from build123d import *

# Parameters (mm, degrees)
SKETCH1_W                       = 82.55
SKETCH1_H                       = 120.65
BOSS_EXTRUDE1_DEPTH             = 69.85
SKETCH2_W                       = 76.2
SKETCH2_H                       = 25.4
CUT_EXTRUDE1_DEPTH              = 107.95
SKETCH3_W                       = 5.08
SKETCH3_H                       = 101.6
CUT_EXTRUDE2_DEPTH              = 8.89
SKETCH4_W                       = 63.5
SKETCH4_H                       = 19.05
CUT_EXTRUDE3_DEPTH              = 83.55
SKETCH5_W                       = 57.15
SKETCH5_H                       = 25.4
CUT_EXTRUDE4_DEPTH              = 121.65
F_40_0_138_DIAMETER_HOLE1_D     = 3.5052
F_40_0_138_DIAMETER_HOLE1_DEPTH = 13.97
BOSS_EXTRUDE2_DEPTH             = 6.35
SKETCH15_W                      = 57.15
SKETCH15_H                      = 88.9
CUT_EXTRUDE5_DEPTH              = 12.7
SKETCH16_W                      = 69.85
SKETCH16_H                      = 6.35
CUT_EXTRUDE6_DEPTH              = 83.55
SKETCH17_R                      = 1.7526
CUT_EXTRUDE7_DEPTH              = 6.35


with BuildPart() as part:
    # Sketch1 → Boss-Extrude1 (new body)
    with BuildSketch(Plane.XY):
        with Locations((0, 79.375)):
            Rectangle(SKETCH1_W, SKETCH1_H)
    extrude(amount=BOSS_EXTRUDE1_DEPTH)

    # Sketch2 → Cut-Extrude1 (cut)
    with BuildSketch(Plane(origin=(0, 139.7, 0), x_dir=(1, 0, 0), z_dir=(0, 1, 0))):
        with Locations((0, -43.18)):
            Rectangle(SKETCH2_W, SKETCH2_H)
    extrude(amount=-CUT_EXTRUDE1_DEPTH, mode=Mode.SUBTRACT)

    # Sketch3 → Cut-Extrude2 (cut)
    with BuildSketch(Plane.XY.offset(69.85)):
        with Locations((30.48, 69.85)):
            Rectangle(SKETCH3_W, SKETCH3_H)
    cut_extrude2 = extrude(amount=-CUT_EXTRUDE2_DEPTH, mode=Mode.SUBTRACT)

    # Mirror1: Cut-Extrude2 across plane
    add(cut_extrude2.mirror(Plane(origin=(0, 0, 0), x_dir=(0, 0, 1), z_dir=(1, 0, 0))), mode=Mode.SUBTRACT)

    # Sketch4 → Cut-Extrude3 (cut, through all)
    with BuildSketch(Plane.ZY.offset(41.275)):
        with Locations((38.1, 130.175)):
            Rectangle(SKETCH4_W, SKETCH4_H)
    extrude(amount=-CUT_EXTRUDE3_DEPTH, mode=Mode.SUBTRACT)

    # Sketch5 → Cut-Extrude4 (cut, through all)
    with BuildSketch(Plane(origin=(0, 139.7, 0), x_dir=(1, 0, 0), z_dir=(0, 1, 0))):
        with Locations((0, -12.7)):
            Rectangle(SKETCH5_W, SKETCH5_H)
    extrude(amount=-CUT_EXTRUDE4_DEPTH, mode=Mode.SUBTRACT)

    # #40 (0.138) Diameter Hole1
    with Locations(Plane.XY.offset(69.85)):
        with Locations((-24.130002345, 92.720002179), (24.129997606, 91.450000321), (8.889995651, 40.650000908)):
            Hole(F_40_0_138_DIAMETER_HOLE1_D / 2, depth=F_40_0_138_DIAMETER_HOLE1_DEPTH)

    # Sketch14 → Boss-Extrude2 (add)
    with BuildSketch(Plane.XZ.offset(-19.05)):
        Polygon((-41.275, 69.85), (-33.02, 69.85), (-33.02, 60.96), (-27.94, 60.96), (-27.94, 69.85), (27.94, 69.85), (27.94, 60.96), (33.02, 60.96), (33.02, 69.85), (41.275, 69.85), (41.275, 0), (28.575, 0), (28.575, 25.4), (-28.575, 25.4), (-28.575, 0), (-41.275, 0), align=None)
    extrude(amount=BOSS_EXTRUDE2_DEPTH)

    # Sketch15 → Cut-Extrude5 (cut)
    with BuildSketch(Plane(origin=(0, 0, 25.4), x_dir=(-1, 0, 0), z_dir=(0, 0, -1))):
        with Locations((0, 57.15)):
            Rectangle(SKETCH15_W, SKETCH15_H)
    extrude(amount=-CUT_EXTRUDE5_DEPTH, mode=Mode.SUBTRACT)

    # Sketch16 → Cut-Extrude6 (cut, through all)
    with BuildSketch(Plane(origin=(41.275, 0, 0), x_dir=(0, 0, -1), z_dir=(1, 0, 0))):
        with Locations((-34.925, 15.875)):
            Rectangle(SKETCH16_W, SKETCH16_H)
    extrude(amount=-CUT_EXTRUDE6_DEPTH, mode=Mode.SUBTRACT)

    # Sketch17 → Cut-Extrude7 (cut)
    with BuildSketch(Plane.XY.offset(6.35)):
        with Locations((-34.925, 133.35)):
            Circle(SKETCH17_R)
    cut_extrude7 = extrude(amount=-CUT_EXTRUDE7_DEPTH, mode=Mode.SUBTRACT)

    # Mirror2: Cut-Extrude7 across plane
    add(cut_extrude7.mirror(Plane(origin=(0, 0, 0), x_dir=(0, 0, 1), z_dir=(1, 0, 0))), mode=Mode.SUBTRACT)


solid = part.part
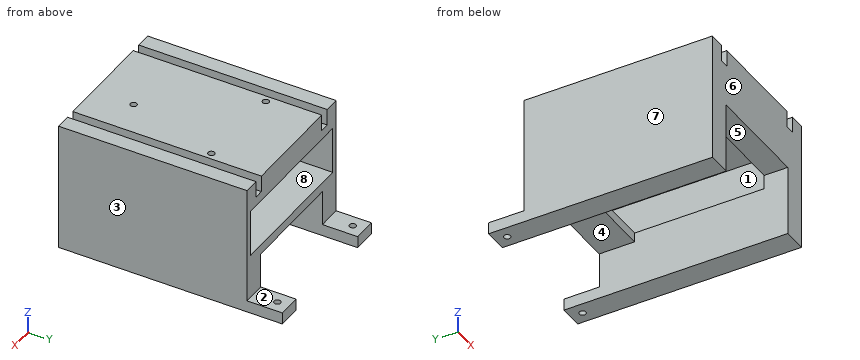
For this review, take the finished solid that the model builds, in its own axes (mm). Face numbers are marked on the shaded views. A direction names the side the tool comes from. Give positions to 0.01 mm unless a question says otherwise; leave off trailing zeros. Order: outer loops, then holes, each group sorted by start corner. A loop starts at its lowest first (then second) coordinate and runs counter-clockwise, first axis right, second up. Notation, with made-up numbers: (46, 89) - (71, 89) arc R25 cw to (71, 102) - close; hole circle Ø2 at (26, 5). An arc over 180 degrees is marked (long way). Answer as a JSON object with one key per item and string values. Group by question number.
Item 1: Take a section at D-D on z = 22.5. Give the boundary of the cut face in (x, y) (3 decimals).
Item 2: Machinability: for the marked faces 1, 2, 3 and 4, which of the approach directions +Z, -Z, +X, -X, +Y, -Y give a long, thin tool a straight path to every point of the face, cutting with its end or side? Answer none if there is none.
Item 3: Take a section at A-A on z = 5. Give the boundary of the cut face in (x, y) (3 decimals).
Item 4: Take a section at B-B on x = 0.5. Give the boundary of the cut face in (y, z), and give its area (3 significant figures).
Item 5: Draft analysis for pull direction X (two halves, no side actions). For the marked faces 5, 6, 7 and 8, state which applies: pulls with the +X half, pulls with the -X half, needs draft (parallel to the pull), parting line crosses it, or undercut.
Item 6: Wall thickness on line 1 along X through (y, z) = (133.35, 4) (3 decimals); line 2 along X through (y, z) = (43, 64.5) (3 decimals); line 3 along Z through (x, y) = (29, 114): over which ranges is each line inside the solid? List them lowest first.
Item 7: Clearance check with flat-ended pins moving along their axes: pin 1 Ø10 at (x, y) = (-32.5, 128.5) entering from +Z; pin 2 Ø19 at (x, z) = (-3.5, 32) entering from +Y; pin 3 Ø1.5 at (x, z) = (-8.5, 27) entering from -Y. State where each tip first meets the part, or that it passes through.
Item 8: Take a section at C-C on y = 40.65. Give the boundary of the cut face in (x, z) (3 decimals), and give its area (3 significant figures).
Reported:
{
 "1": {"outline": "(-41.275, 19.05) - (-28.575, 19.05) - (-28.575, 120.65) - (-41.275, 120.65) - close; (28.575, 19.05) - (41.275, 19.05) - (41.275, 120.65) - (28.575, 120.65) - close"},
 "2": {"face 1": "+Y", "face 2": "+Z, +X, -X, +Y", "face 3": "+Z, -Z, +X, +Y, -Y", "face 4": "-Z, +Y, -Y"},
 "3": {"outline": "(-41.275, 19.05) - (-28.575, 19.05) - (-28.575, 139.7) - (-41.275, 139.7) - close; (28.575, 19.05) - (41.275, 19.05) - (41.275, 139.7) - (28.575, 139.7) - close; hole circle Ø3.505 at (-34.925, 133.35); hole circle Ø3.505 at (34.925, 133.35)"},
 "4": {"outline": "(19.05, 38.1) - (31.75, 38.1) - (31.75, 55.88) - (120.65, 55.88) - (120.65, 69.85) - (19.05, 69.85) - close; (101.6, 25.4) - (120.65, 25.4) - (120.65, 30.48) - (101.6, 30.48) - close", "area": "1,740 mm^2"},
 "5": {"face 5": "undercut", "face 6": "needs draft", "face 7": "pulls with the -X half", "face 8": "undercut"},
 "6": {"line 1": "-41.275 to -36.678, -33.172 to -28.575, 28.575 to 33.172, 36.678 to 41.275", "line 2": "-41.275 to -33.02, -27.94 to 27.94, 33.02 to 41.275", "line 3": "0 to 30.48, 55.88 to 60.96"},
 "7": {"pin 1": "z = 6.35", "pin 2": "y = 120.65", "pin 3": "y = 101.6"},
 "8": {"outline": "(-41.275, 0) - (-28.575, 0) - (-28.575, 30.48) - (-38.1, 30.48) - (-38.1, 55.88) - (7.137, 55.88) - (7.137, 69.85) - (-27.94, 69.85) - (-27.94, 60.96) - (-33.02, 60.96) - (-33.02, 69.85) - (-41.275, 69.85) - close; (10.643, 55.88) - (38.1, 55.88) - (38.1, 30.48) - (28.575, 30.48) - (28.575, 0) - (41.275, 0) - (41.275, 69.85) - (33.02, 69.85) - (33.02, 60.96) - (27.94, 60.96) - (27.94, 69.85) - (10.643, 69.85) - close", "area": "1,950 mm^2"}
}
